Source: CAD feature listing. Evaluate the final solid. Frame: model axes, mm. Coordinates: 2 decimals unless noted, no trailing zeros. Order: outer loops, then holes, each group sorted by start corner. A loop starts at its lowest first (then second) coordinate and runs counter-clockwise, first axis right, second up.
Item 1: Section A-A on z = 50. Return the cut outline in (x, y).
Item 2: Contact query for flat-ended pins moving along their axis: P1, Ø12, axis at y = 231.5, z = 32, coming from the +X side; P2, Ø1, axis at y = 49, z = 18.5, coming from the +X side; P3, Ø2, axis at y = 144, z = 49.5, coming from the -X side; P4, Ø3, axis at x = 47.5, y = 198, coming from the -Z side. Output: stop coordinate, or through.
Item 3: Section B-B on x = 54.5. Return the cut outline in (y, z), then the cut area to 3 significant figures.
Item 4: Section C-C on y = 115.5. Return the cut outline in (x, z).
Item 5: Ray query, line 1 (X direction, y = -82, z = 73); line 2 (Y direction, x = 87.5, z = 29); line 3 (Y direction, x = -87.5, z = 60). Return the intervals inside material, ascending.
from build123d import *

# Parameters (mm, degrees)
F1_DEPTH = 80


with BuildPart() as f1:
    # F0 (on Top) → F1 (new body)
    with BuildSketch(Plane.XY):
        Polygon((-138.8081118726, 243.2102153142), (-219.5454731322, 94.7753002802), (-171.6760737886, -67.273970347), (-23.2411587546, -148.0113316066), (138.8081118726, -100.141932263), (219.5454731322, 48.292982771), (171.6760737886, 210.3422533982), (23.2411587546, 291.0796146578), align=None)
        with BuildLine():
            Line((-79.5, 183.2811294774), (0, 183.2811294774))
            Line((0, 183.2811294774), (79.5, 183.2811294774))
            ThreePointArc((79.5, 183.2811294774), (87.5, 191.2811294774), (95.5, 183.2811294774))
            ThreePointArc((95.5, 183.2811294774), (93.4912722212, 177.9797469057), (88.473835707, 175.3406229435))
            Line((88.473835707, 175.3406229435), (119.026164293, -73.7783639886))
            ThreePointArc((119.026164293, -73.7783639886), (125.3013825717, -75.7275983014), (128, -81.7188705226))
            ThreePointArc((128, -81.7188705226), (120, -89.7188705226), (112, -81.7188705226))
            Line((112, -81.7188705226), (0, -81.7188705226))
            Line((0, -81.7188705226), (-112, -81.7188705226))
            ThreePointArc((-112, -81.7188705226), (-125.9912722212, -87.0202530943), (-119.026164293, -73.7783639886))
            Line((-119.026164293, -73.7783639886), (-88.473835707, 175.3406229435))
            ThreePointArc((-88.473835707, 175.3406229435), (-92.8013825717, 189.2724016986), (-79.5, 183.2811294774))
        make_face(mode=Mode.SUBTRACT)
        with BuildLine():
            Line((82.567931818, 176.9823436064), (0, 71.5341415256))
            Line((0, 71.5341415256), (115.067931818, -75.4200846516))
            ThreePointArc((115.067931818, -75.4200846516), (116.9350796307, -74.3292654499), (119.026164293, -73.7783639886))
            Line((119.026164293, -73.7783639886), (88.473835707, 175.3406229435))
            ThreePointArc((88.473835707, 175.3406229435), (85.3574051327, 175.5733874452), (82.567931818, 176.9823436064))
        make_face()
        with BuildLine():
            Line((115.067931818, -75.4200846516), (0, 71.5341415256))
            Line((0, 71.5341415256), (0, -81.7188705226))
            Line((0, -81.7188705226), (112, -81.7188705226))
            ThreePointArc((112, -81.7188705226), (112.8077630234, -78.2157680017), (115.067931818, -75.4200846516))
        make_face()
        with BuildLine():
            Line((0, -81.7188705226), (0, 71.5341415256))
            Line((0, 71.5341415256), (-115.067931818, -75.4200846516))
            ThreePointArc((-115.067931818, -75.4200846516), (-112.8077630234, -78.2157680017), (-112, -81.7188705226))
            Line((-112, -81.7188705226), (0, -81.7188705226))
        make_face()
        with BuildLine():
            Line((-115.067931818, -75.4200846516), (0, 71.5341415256))
            Line((0, 71.5341415256), (-82.567931818, 176.9823436064))
            ThreePointArc((-82.567931818, 176.9823436064), (-85.3574051327, 175.5733874452), (-88.473835707, 175.3406229435))
            Line((-88.473835707, 175.3406229435), (-119.026164293, -73.7783639886))
            ThreePointArc((-119.026164293, -73.7783639886), (-116.9350796307, -74.3292654499), (-115.067931818, -75.4200846516))
        make_face()
        with BuildLine():
            Line((79.5, 183.2811294774), (0, 183.2811294774))
            Line((0, 183.2811294774), (0, 71.5341415256))
            Line((0, 71.5341415256), (82.567931818, 176.9823436064))
            ThreePointArc((82.567931818, 176.9823436064), (80.3077630234, 179.7780269565), (79.5, 183.2811294774))
        make_face()
        with BuildLine():
            Line((0, 71.5341415256), (0, 183.2811294774))
            Line((0, 183.2811294774), (-79.5, 183.2811294774))
            ThreePointArc((-79.5, 183.2811294774), (-80.3077630234, 179.7780269565), (-82.567931818, 176.9823436064))
            Line((-82.567931818, 176.9823436064), (0, 71.5341415256))
        make_face()
    extrude(amount=F1_DEPTH)


solid = f1.part
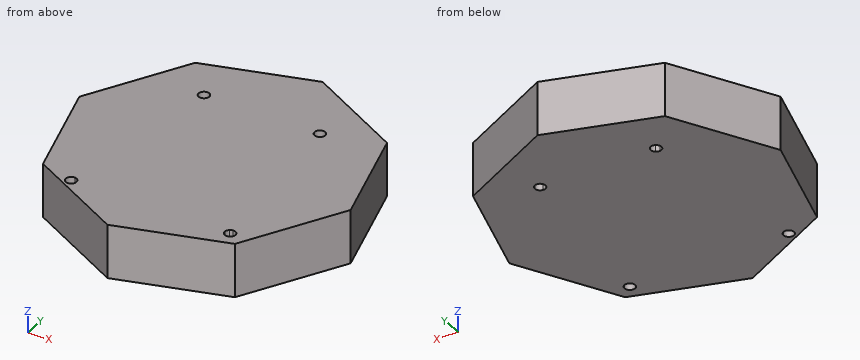
Answer list:
1. outline: (-219.55, 94.78) - (-171.68, -67.27) - (-23.24, -148.01) - (138.81, -100.14) - (219.55, 48.29) - (171.68, 210.34) - (23.24, 291.08) - (-138.81, 243.21) - close; hole circle Ø16 at (-120, -81.72); hole circle Ø16 at (-87.5, 183.28); hole circle Ø16 at (87.5, 183.28); hole circle Ø16 at (120, -81.72)
2. P1: stops at x = 143.81
2. P2: stops at x = 219.48
2. P3: stops at x = -193.31
2. P4: stops at z = 0
3. outline: (-125.05, 0) - (274.08, 0) - (274.08, 80) - (-125.05, 80) - close
3. area: 31,900 mm2
4. outline: (-208.27, 0) - (199.69, 0) - (199.69, 80) - (-208.27, 80) - close
5. line 1: x = -144.6 to -128, -112 to 112, 128 to 148.68
5. line 2: y = -115.3 to 175.28, 191.28 to 256.13
5. line 3: y = -113.06 to 175.28, 191.28 to 258.37
